Autodesk Inventor part; units mm, degrees
ref_plane "Work Plane1" through (0, 0, -16) normal (0, 0, 1) x (1, 0, 0)
ref_plane "Work Plane2" through (0, 0, 16) normal (0, 0, 1) x (1, 0, 0)
ref_plane "Work Plane3" through (-16, 0, 0) normal (1, 0, 0) x (0, 1, 0)
sketch "Body" plane through (0, 0, 0) normal (0, 1, 0) x (-1, 0, 0)
  circle A0 centre (0, 0) radius 5
  circle A1 centre (0, 0) radius 19
  line L0 (0, -19) -> (128.5, -19)
  line L1 (128.5, -19) -> (128.5, 19)
  line L2 (128.5, 19) -> (0, 19)
  line L3 (0, 19) -> (0, -19)
  line L4 (158, 0) -> (-48.5, 0) construction
  line L5 (0, -26.6) -> (0, 26.6) construction
  line L6 (-19, 0) -> (128.5, 0)
  point P0 (0, 0)
  dimension "d0" = 10
  dimension "d1" = 38
  dimension "d2" = 38
  dimension "d3" = 128.5
revolve "BodyFeature" add sketch "Body" angle 360 about axis through (19, 0, 0) along (-1, 0, 0) picked at (14.1328, -1.7802) picked at (1.7623, -2.8047) picked at (-1.7802, -14.1328) picked at (-0.3709, -3.2915) contours L6 A1 L3 A0 | A0 L3 L6 | L3 A1 L6 A0 | A0 L6 L3 | L6 L1 L0 A1
ref_plane "Work Plane1" through (0, 0, -16) normal (0, 0, 1) x (1, 0, 0)
ref_plane "Work Plane2" through (0, 0, 16) normal (0, 0, 1) x (1, 0, 0)
sketch "Sketch2" plane through (0, 0, -16) normal (0, 0, 1) x (1, 0, 0)
  arc A0 (0, -19) -> (0, 19) centre (0, 0) ccw
  arc A1 (0, -10) -> (0, 10) centre (0, 0) ccw
  line L0 (0, -19) -> (0, -10) construction
  line L1 (0, 19) -> (0, -19) construction
  line L2 (0, -10) -> (-14, -10)
  line L3 (-14, -10) -> (-14, 10)
  line L4 (-14, 10) -> (0, 10)
  line L5 (-14, 10) -> (-14, -10)
  dimension "d7" = 10
  dimension "d8" = 14
extrude "Extrusion1" cut sketch "Sketch2" against normal through all
mirror "Mirror1" about plane through (0, 0, 0) normal (0, 0, 1) of "Extrusion1"
sketch "Sketch3" plane through (0, 0, -16) normal (0, 0, -1) x (-1, 0, 0)
  circle A0 centre (0, 0) radius 5
  dimension "d11" = 10
extrude "Extrusion2" cut sketch "Sketch3" against normal through all
fillet "Fillet1" radius 1 1 edges at (-14, 0, -16)
ref_plane "Work Plane3" through (-16, 0, 0) normal (1, 0, 0) x (0, 1, 0)
sketch "Sketch4" plane through (-16, 0, 0) normal (1, 0, 0) x (0, 1, 0)
  circle A0 centre (0, 0) radius 19
  circle A1 centre (0, 0) radius 18.75
  dimension "d16" = 0.25
extrude "Extrusion3" cut sketch "Sketch4" along normal mid plane 0.25
ref_plane "Work Plane4" through (-118.5, 0, 0) normal (-1, 0, 0) x (0, 0, 1)
sketch "Sketch5" plane through (-118.5, 0, 0) normal (-1, 0, 0) x (0, 0, 1)
  circle A0 centre (0, 0) radius 19
  circle A1 centre (0, 0) radius 18.75
  dimension "d20" = 0.25
extrude "Extrusion4" cut sketch "Sketch5" along normal mid plane 0.25
chamfer "Chamfer1" distance 1 angle 45 1 edges at (-128.5, 0, 19)
properties part number "ANT-38-Body"
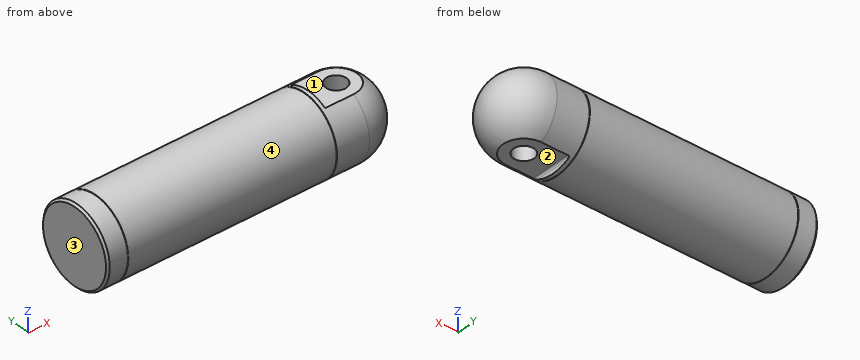
Geometry check sheet. Reference: the model listing, model coordinates, mm. Face numbers are marked on the shaded views. Coordinates: 2 decimals unless noted, no trailing zeros. Order: outer loops, then holes, each group sorted by start corner. A loop starts at its lowest first (then second) coordinate and runs counter-clockwise, first axis right, second up. Notation, with made-up numbers: M 18.5,-9 L 60.5,-9 A34 ccw 60.5,29 Z; hole C 60.25,17.5 d9. An arc over 180 degrees is marked long. Answer as a JSON object with one key per item and string values.
Q1. Cross-section at C-C on x = -8.5. Record the cut outline in (y, z), and give its area (3 significant figures).
Results are:
{"outline": "M -10,-16.16 L -10,-16 L 10,-16 L 10,-16.16 A19 ccw 10,16.16 L 10,16 L -10,16 L -10,16.16 A19 ccw Z", "area": "1,050 mm²"}
Q2. Cross-section at D-D on x = -30.5. Record the cut outline in (y, z).
Results are:
{"outline": "C 0,0 d38"}
Q3. Scan lines: line 1 (Y direction, x = 0, z = 3); line 2 (Z direction, x = -55, y = -1); line 3 (Y direction, x = -24, z = -6). Record each from-to range of solid material in increasing order.
Results are:
{"line 1": "y = -18.76 to -5, 5 to 18.76", "line 2": "z = -18.97 to 18.97", "line 3": "y = -18.03 to 18.03"}
Q4. Release check for a two-part mould opening along X. For the marked faces 1, 2, 3 and 4 record: released by +X, released by -X, zero draft, split by the parting line, or undercut.
Results are:
{"face 1": "undercut", "face 2": "undercut", "face 3": "released by -X", "face 4": "zero draft"}
Q5. Depth check by flat-ended pin: pin 1 Ø5 at (x, z) = (-102.5, 14) entering from -Y; pin 2 Ø1.5 at (x, z) = (-28, -11) entering from -Y; pin 3 Ø0.6 at (y, z) = (4, -18) entering from +X; pin 4 Ø2 at (x, y) = (-86.5, -0.5) entering from +Z. Enter the tip coordinate at first touch or a pass-through.
Results are:
{"pin 1": "stops at y = -15.12", "pin 2": "stops at y = -16", "pin 3": "stops at x = -14", "pin 4": "stops at z = 19"}
Q6. Cross-section at B-B on z = 0. Record the cut outline in (x, y) (3 decimals).
Results are:
{"outline": "M -128.5,-18 L -127.5,-19 L -118.625,-19 L -118.625,-18.75 L -118.375,-18.75 L -118.375,-19 L -16.125,-19 L -16.125,-18.75 L -15.875,-18.75 L -15.875,-19 L 0,-19 A19 ccw 0,19 L -15.875,19 L -15.875,18.75 L -16.125,18.75 L -16.125,19 L -118.375,19 L -118.375,18.75 L -118.625,18.75 L -118.625,19 L -127.5,19 L -128.5,18 Z; hole C 0,0 d10"}
